Drawing for the job (mm, zero at the part's lowest x, y, z). Round coordinates to 2 decimals unless told otherwise and drop trailing zeros. Write each loop counter-clockwise with the first axis right and the second up, starting at its lowest first coordinate (ties: lowest second). Pieces come first, ordered by that corner, then holes. Notation, with made-up numbers: M 77,47 L 97,47 A26 ccw 97,78 Z; hole C 30.25,-4 d5. An arc over 180 degrees is marked long. Use a Markdown table: item, result. Add a question column.
1) Slice it at A-A on z = 86.5. Write the cut outline in (x, y), plus the area to 3 significant figures.
2) Wall check: probe 1 along X at (y, z) = (113.5, 151); probe 2 along X at (y, z) = (171, 147); probe 3 along Z at (x, y) = (105, 244). Give the ranges that are in metal, low to high.
3) Drop flat-ended pins along their axis: P1, Ø4, axis at y = 84.5, z = 87.5, coming from the +X side; P2, Ø5, axis at x = 73, y = 154, coming from the +Z side; P3, Ø8, axis at x = 182, z = 185, coming from the -Y side. Give the stop position or say it passes through.
4) Slice it at B-B on x = 101.5. Write the cut outline in (y, z), plus the area to 3 significant figures.
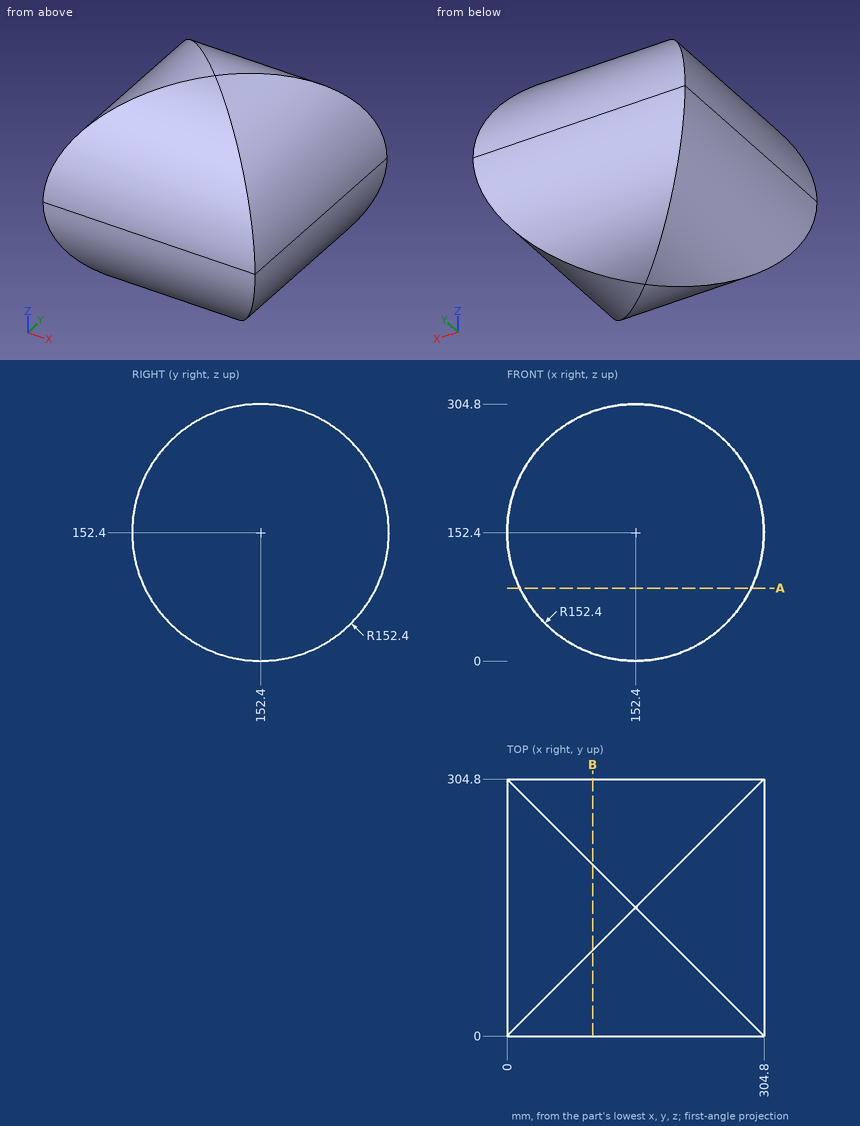
Entries:
| question | item | result |
|---|---|---|
| 1 | outline | M 14.98,14.98 L 289.82,14.98 L 289.82,289.82 L 14.98,289.82 Z |
| 1 | area | 75,500 mm^2 |
| 2 | probe 1 | x = 0.01 to 304.79 |
| 2 | probe 2 | x = 0.1 to 304.7 |
| 2 | probe 3 | z = 30.6 to 274.2 |
| 3 | P1 | stops at x = 291.21 |
| 3 | P2 | stops at z = 283.98 |
| 3 | P3 | stops at y = 2.71 |
| 4 | outline | M 101.5,8.75 L 203.3,8.75 A152.4 ccw 203.3,296.05 L 101.5,296.05 A152.4 ccw Z |
| 4 | area | 71,800 mm^2 |
